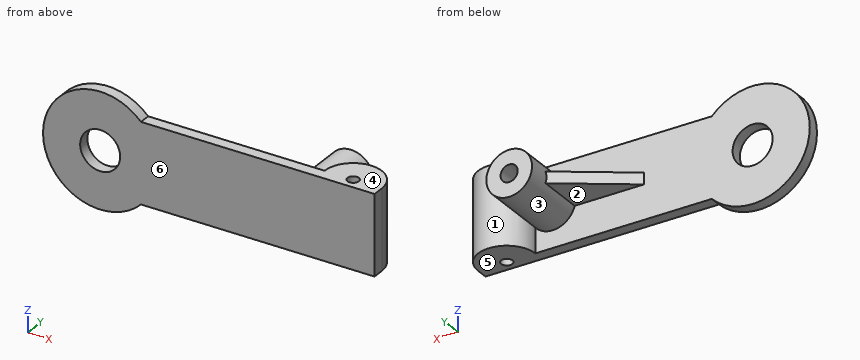
```python
from build123d import *

# Parameters (mm, degrees)
SKETCH2_R           = 17.5
BOSS_EXTRUDE1_DEPTH = 10
SKETCH3_R           = 20
SKETCH3_R_2         = 7.5
BOSS_EXTRUDE2_DEPTH = 60
BOSS_EXTRUDE7_DEPTH = 5
BOSS_EXTRUDE8_DEPTH = 35
SKETCH5_R           = 5
CUT_EXTRUDE1_DEPTH  = 70


with BuildPart() as part:
    # Sketch2 → Boss-Extrude1 (new body)
    with BuildSketch(Plane(origin=(0, 0, 0), x_dir=(1, 0, 0), z_dir=(0, 1, 0))):
        with BuildLine():
            Line((0, -35), (-204.292857857, -35))
            ThreePointArc((-204.292857857, -35), (-290, 0), (-204.292857857, 35))
            Line((-204.292857857, 35), (0, 35))
            Line((0, 35), (0, -35))
        make_face()
        with Locations(Location((-240, 0, 0), (0, 0, 270))):
            Circle(SKETCH2_R, mode=Mode.SUBTRACT)
    extrude(amount=BOSS_EXTRUDE1_DEPTH)

    # Sketch3 → Boss-Extrude2 (add)
    with BuildSketch(Plane(origin=(0, 10, 0), x_dir=(1, 0, 0), z_dir=(0, 1, 0))):
        with Locations(Location((-65, 0, 0), (0, 0, 270))):
            Circle(SKETCH3_R)
        with Locations(Location((-65, 0, 0), (0, 0, 270))):
            Circle(SKETCH3_R_2, mode=Mode.SUBTRACT)
    extrude(amount=BOSS_EXTRUDE2_DEPTH)

    # Sketch4 → Boss-Extrude7 (add, symmetric)
    with BuildSketch(Plane.XY):
        Polygon((-145, 10), (-81.055755384, 10), (-81.055755384, 52.629496411), align=None)
    extrude(amount=BOSS_EXTRUDE7_DEPTH, both=True)

    # Sketch4_6 → Boss-Extrude8 (add, symmetric)
    with BuildSketch(Plane.XY):
        with BuildLine():
            Line((-50, 10), (0, 10))
            ThreePointArc((0, 10), (-25, 35), (-50, 10))
        make_face()
    extrude(amount=BOSS_EXTRUDE8_DEPTH, both=True)

    # Sketch5 → Cut-Extrude1 (cut)
    with BuildSketch(Plane.XY.offset(35)):
        with Locations((-25, 10)):
            Circle(SKETCH5_R)
    extrude(amount=-CUT_EXTRUDE1_DEPTH, mode=Mode.SUBTRACT)


solid = part.part
```
Check sheet for the modelled part. Datum: model origin and axes. Units: mm. Face numbers are marked on the shaded views. A direction names the side the tool comes from. Round coordinates to 2 decimals unless told otherwise and drop trailing zeros. Write each loop counter-clockwise with the first axis right and the second up, starting at its lowest first coordinate (ties: lowest second). Pieces come first, ordered by that corner, then holes. Notation, with made-up numbers: (-1, 55.5) -> (36, 55.5) arc R23 ccw to (36, 75.5) -> close; hole circle Ø8 at (-29, 42). An arc over 180 degrees is marked (long way). Put each result on its own line as item: value.
(1) Sectioned sample at A-A (x = -240). Enter the section's corners in (y, z), plus the area to 3 significant figures.
Values found:
outline: (0, -50) -> (10, -50) -> (10, -17.5) -> (0, -17.5) -> close; (0, 17.5) -> (10, 17.5) -> (10, 50) -> (0, 50) -> close
area: 650 mm^2
(2) Sectioned sample at D-D (x = -104). Enter the section's corners in (y, z), plus the area to 3 significant figures.
Values found:
outline: (0, -35) -> (10, -35) -> (10, -5) -> (37.33, -5) -> (37.33, 5) -> (10, 5) -> (10, 35) -> (0, 35) -> close
area: 973 mm^2
(3) Go/stop test with flat-tipped pins: pin 1 Ø12 at (x, y) = (-118.5, 25.5) entering from +Z; pin 2 Ø3 at (x, z) = (-104.5, 26) entering from -Y; pin 3 Ø13 at (x, y) = (-25, 10) entering from -Z; pin 4 Ø3 at (x, z) = (-41.5, 14) entering from +Y. Record where each tip stops, or that it passes through.
Values found:
pin 1: stops at z = 5
pin 2: stops at y = 0
pin 3: stops at z = -35
pin 4: stops at y = 30
(4) Mould release check, pull along X, two halves, no side actions. Record for the marked faces 1, 2 and 3: released by +X, released by -X, zero draft, split by the parting line, or undercut.
Values found:
face 1: undercut
face 2: zero draft
face 3: undercut
(5) Sectioned sample at C-C (x = -25). Enter the section's corners in (y, z), plus the area to 3 significant figures.
Values found:
outline: (0, -35) -> (5, -35) -> (5, 35) -> (0, 35) -> close; (15, -35) -> (35, -35) -> (35, 35) -> (15, 35) -> close
area: 1,750 mm^2
(6) Sectioned sample at B-B (y = 40). Enter the section's corners in (x, z).
Values found:
outline: (-100, -5) -> (-84.36, -5) arc R20 ccw (long way) to (-84.36, 5) -> (-100, 5) -> close; hole circle Ø15 at (-65, 0)
(7) Tool access check on the marked faces 4, 5 and 6. Record the directions out of +Z, -Z, +X, -X, +Y, -Y that give a thin tool (end or side, any length) a straight path to the whole face; none if there is none.
Values found:
face 4: +Z, +X, +Y, -Y
face 5: -Z, +X, +Y, -Y
face 6: +Z, -Z, +X, -X, -Y
(8) Material ranges on line 1 (X direction, y = 32, z = 1); line 2 (Z direction, x = -87, y = 33.5); line 3 (X direction, y = 23, z = -14), recorded low to high.
Values found:
line 1: x = -112 to -72.43, -57.57 to -45.03, -36.87 to -13.13
line 2: z = -5 to 5
line 3: x = -79.28 to -50.72, -46.35 to -3.65
